Read the model definition and answer for the solid it produces. Units are mm, in the model's axes. Face numbers are marked on the shaded views. A direction names the side the tool comes from. Round coordinates to 2 decimals unless told otherwise and drop trailing zeros. Order: outer loops, then holes, each group sorted by start corner. A loop starts at its lowest first (then second) coordinate and runs counter-clockwise, first axis right, second up. Notation, with made-up numbers: (-0.75, 6.5) -> (49.25, 6.5) arc R29 ccw to (49.25, 40.5) -> close; hole circle Ø3 at (74, -6). An arc over 180 degrees is marked (long way). One line per item, written item: value. Start each with the question number.
1. Section D-D (z = 47.5) is taken. Give the vertices of the cut face in (x, y), then the cut area to 3 significant figures.
2. The mould has two halves that part along Z. Classify the marked faces 1, 2 and 3: released by +Z, released by -Z, zero draft, split by the parting line, or undercut.
3. Consider line 1 (X direction, y = 181, z = 57.5); line 2 (Z direction, x = 78.75, y = 182.1); line 3 (Y direction, x = 78, z = 52). Determine where each line is inside the solid, lowest interval first.
4. Flat-ended cylindrical pins translate along their axes: pin 1 Ø4 at (x, y) = (79.5, 188) entering from +Z; pin 2 Ø4 at (x, z) = (77, 55.5) entering from -Y; pin 3 Ø1.5 at (x, y) = (77.5, 186) entering from -Z. Find the tip coordinate at first contact, or state that the pin passes through.
5. Section C-C (x = 81.75) is taken. Give the vertices of the cut face in (y, z).
6. For the marked faces 4 and 5, determine the directions among +Z, -Z, +X, -X, +Y, -Y from which every point of the face is accessible in a straight line to the end or side of a thin tool.
7. Section A-A (z = 51.18) is taken. Give the vertices of the cut face in (x, y), then the cut area to 3 significant figures.
8. Section B-B (y = 182.1) is taken. Give the vertices of the cut face in (x, z), then the cut area to 3 significant figures.
from build123d import *

# Parameters (mm, degrees)
CYLINDER286_R          = 2.5
CYLINDER286_DEPTH      = 14.5
CYLINDER289_R          = 6
CYLINDER289_DEPTH      = 6.5
CYLINDER288_R          = 9
CYLINDER288_DEPTH      = 1
CYLINDER287_R          = 9
CYLINDER287_DEPTH      = 1
CUT203_ROLL_ANGLE      = 90
CUT203_PLACEMENT_ANGLE = 90


with BuildPart() as cylinder286:
    # Cylinder286 → Cylinder286 (new body)
    with BuildSketch(Plane.XY.offset(-2.4)):
        Circle(CYLINDER286_R)
    extrude(amount=CYLINDER286_DEPTH)


with BuildPart() as cylinder289:
    # Cylinder289 → Cylinder289 (new body)
    with BuildSketch(Plane.XY.offset(1)):
        Circle(CYLINDER289_R)
    extrude(amount=CYLINDER289_DEPTH)


with BuildPart() as cylinder288:
    # Cylinder288 → Cylinder288 (new body)
    with BuildSketch(Plane.XY.offset(7.5)):
        Circle(CYLINDER288_R)
    extrude(amount=CYLINDER288_DEPTH)


with BuildPart() as cut203:
    # Cylinder287 → Cylinder287 (new body)
    with BuildSketch(Plane.XY):
        Circle(CYLINDER287_R)
    extrude(amount=CYLINDER287_DEPTH)

    # Fusion109: union Cylinder289, Cylinder288
    add(cylinder289.part)
    add(cylinder288.part)

    # Cut203: cut Cylinder286
    add(cylinder286.part, mode=Mode.SUBTRACT)


with BuildPart() as cut203_1:
    # Cut203 roll: moved
    add(cut203.part.rotate(Axis((0, 0, 0), (1, 0, 0)), CUT203_ROLL_ANGLE))


with BuildPart() as cut203_2:
    # Cut203 placement: moved
    add(cut203_1.part.moved(Location((73.8, 182.1, 51.18))).rotate(Axis((73.8, 182.1, 51.18), (0, 0, 1)), CUT203_PLACEMENT_ANGLE))


solid = cut203_2.part
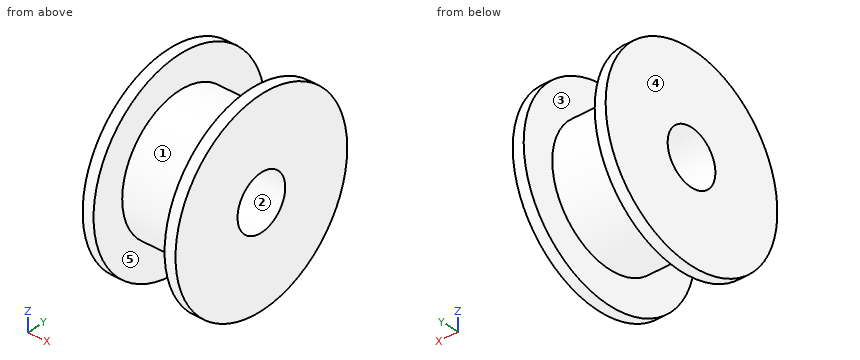
Answer:
1. outline: (73.8, 173.89) -> (74.8, 173.89) -> (74.8, 177.36) -> (81.3, 177.36) -> (81.3, 173.89) -> (82.3, 173.89) -> (82.3, 190.31) -> (81.3, 190.31) -> (81.3, 186.84) -> (74.8, 186.84) -> (74.8, 190.31) -> (73.8, 190.31) -> close
1. area: 94.5 mm^2
2. face 1: split by the parting line
2. face 2: undercut
2. face 3: zero draft
3. line 1: 73.8 to 74.8, 81.3 to 82.3
3. line 2: 45.18 to 48.68, 53.68 to 57.18
3. line 3: 176.16 to 179.74, 184.46 to 188.04
4. pin 1: z = 58.64
4. pin 2: y = 176.57
4. pin 3: z = 46.07
5. outline: circle Ø18 at (182.1, 51.18); hole circle Ø5 at (182.1, 51.18)
6. face 4: +Z, -Z, -X, +Y, -Y
6. face 5: none
7. outline: (73.8, 173.1) -> (74.8, 173.1) -> (74.8, 176.1) -> (81.3, 176.1) -> (81.3, 173.1) -> (82.3, 173.1) -> (82.3, 179.6) -> (73.8, 179.6) -> close; (73.8, 184.6) -> (82.3, 184.6) -> (82.3, 191.1) -> (81.3, 191.1) -> (81.3, 188.1) -> (74.8, 188.1) -> (74.8, 191.1) -> (73.8, 191.1) -> close
7. area: 71.5 mm^2
8. outline: (73.8, 42.18) -> (74.8, 42.18) -> (74.8, 45.18) -> (81.3, 45.18) -> (81.3, 42.18) -> (82.3, 42.18) -> (82.3, 48.68) -> (73.8, 48.68) -> close; (73.8, 53.68) -> (82.3, 53.68) -> (82.3, 60.18) -> (81.3, 60.18) -> (81.3, 57.18) -> (74.8, 57.18) -> (74.8, 60.18) -> (73.8, 60.18) -> close
8. area: 71.5 mm^2
